from build123d import *

# Parameters (mm, degrees)
BOSS_EXTRUDE2_DEPTH   = 12.7
BOSS_EXTRUDE2_2_DEPTH = 12.7
SKETCH2_7_W           = 239.064376672
SKETCH2_7_H           = 153.94029831
BOSS_EXTRUDE3_DEPTH   = 12.7
SKETCH2_8_R           = 5.08
SKETCH2_8_R_2         = 3.81
BOSS_EXTRUDE4_DEPTH   = 50.8


with BuildPart() as part:
    # Sketch2 → Boss-Extrude2 (new body)
    with BuildSketch(Plane.XY):
        Polygon((-103.331182916, 71.628), (103.331182916, 71.628), (98.251182916, 76.708), (-98.251182916, 76.708), align=None)
    extrude(amount=BOSS_EXTRUDE2_DEPTH)



with BuildPart() as body_2:
    # Sketch2 → Boss-Extrude2 2 (new body)
    with BuildSketch(Plane.XY):
        Polygon((103.331182916, 107.188), (98.251182916, 102.108), (-98.251182916, 102.108), (-103.331182916, 107.188), align=None)
    extrude(amount=BOSS_EXTRUDE2_2_DEPTH)


with BuildPart() as part_1:
    add(part.part)

    add(body_2.part)  # Boss-Extrude3 merges body 2
    # Sketch2_7 → Boss-Extrude3 (add)
    with BuildSketch(Plane.XY):
        with Locations((0, 44.704)):
            Rectangle(SKETCH2_7_W, SKETCH2_7_H)
    extrude(amount=-BOSS_EXTRUDE3_DEPTH)

    # Sketch2_8 → Boss-Extrude4 (add)
    with BuildSketch(Plane.XY):
        with Locations((21.333013583, 41.868396572)):
            Circle(SKETCH2_8_R)
        Circle(SKETCH2_8_R_2)
    extrude(amount=BOSS_EXTRUDE4_DEPTH)


solid = part_1.part
Geometry check sheet. Reference: the model listing, model coordinates, mm. A direction names the side the tool comes from. Round coordinates to 2 decimals unless told otherwise and drop trailing zeros. Loops run counter-clockwise (first coordinate to the right, second up) from the corner with the lowest first, then second, coordinate; pieces in that order, holes last. Notation, with made-up numbers: (15, 10) -> (45, 10) arc R19 ccw to (45, 16) -> close; hole circle Ø1 at (-26, 40.5). An arc over 180 degrees is marked (long way). Answer as a JSON object with one key per item and string values. Group by question number.
Item 1: Cross-section at A-A, the plane x = -86. Record the cut outline in (y, z).
Item 2: Cross-section at B-B, the plane y = 0. Record the cut outline in (x, z), plus the area to 3 significant figures.
Item 3: Set-up check for faces 1 (the face through (100.83, 74.13, 6.26)), 2 (the face through (-100.756, 104.612, 6.261)), 3 (the face through (-1, 74, 12.7)), 4 (the face through (-0.83, -3.72, 25.04)), 5 (the face through (-1, 71.628, 6)): record each of +Z, -Z, +X, -X, +Y, -Y from which the full face is reachable in a straight line by a thin tool's end or side.
Item 4: Release check for a two-part mould opening along Y. For faces 6 (the face through (1, 105, 12.7)), 7 (the face through (100.827, 104.684, 6.261)), 8 (the face through (-2, -32.266, -6)) record: pulls with the +Y half, pulls with the -Y half, needs draft (parallel to the pull), parting line crosses it, or undercut.
Item 5: Cross-section at D-D, the plane x = 0. Record the cut outline in (y, z).
Item 6: Cross-section at C-C, the plane z = 6.5. Record the cut outline in (x, y).
Item 7: Depth check by flat-ended pin: pin 1 Ø6.5 at (x, z) = (4.5, 6) entering from +Y; pin 2 Ø6.5 at (x, z) = (25.5, 8) entering from -Y; pin 3 Ø2.5 at (x, y) = (-8, 105.5) entering from +Z; pin 4 Ø6 at (y, z) = (-7, 28) entering from -X. Enter the tip coordinate at first touch or a pass-through.
Item 8: Thickness scan on line 1 along Y through (x, z) = (-3.5, 2); line 2 along X through (y, z) = (0.5, 32); line 3 along Z through (x, y) = (92, 47). Record the ranges inside material, lowest first.
Determined:
{
 "1": {"outline": "(-32.27, -12.7) -> (121.67, -12.7) -> (121.67, 0) -> (107.19, 0) -> (107.19, 12.7) -> (102.11, 12.7) -> (102.11, 0) -> (76.71, 0) -> (76.71, 12.7) -> (71.63, 12.7) -> (71.63, 0) -> (-32.27, 0) -> close"},
 "2": {"outline": "(-119.53, -12.7) -> (119.53, -12.7) -> (119.53, 0) -> (3.81, 0) -> (3.81, 50.8) -> (-3.81, 50.8) -> (-3.81, 0) -> (-119.53, 0) -> close", "area": "3,420 mm²"},
 "3": {"face 1": "+Z, +X", "face 2": "+Z, -X", "face 3": "+Z, +X, -X, +Y", "face 4": "+Z", "face 5": "+Z, +X, -X"},
 "4": {"face 6": "needs draft", "face 7": "undercut", "face 8": "pulls with the -Y half"},
 "5": {"outline": "(-32.27, -12.7) -> (121.67, -12.7) -> (121.67, 0) -> (107.19, 0) -> (107.19, 12.7) -> (102.11, 12.7) -> (102.11, 0) -> (76.71, 0) -> (76.71, 12.7) -> (71.63, 12.7) -> (71.63, 0) -> (3.81, 0) -> (3.81, 50.8) -> (-3.81, 50.8) -> (-3.81, 0) -> (-32.27, 0) -> close"},
 "6": {"outline": "(-103.33, 71.63) -> (103.33, 71.63) -> (98.25, 76.71) -> (-98.25, 76.71) -> close; (-103.33, 107.19) -> (-98.25, 102.11) -> (98.25, 102.11) -> (103.33, 107.19) -> close; circle Ø7.62 at (0, 0); circle Ø10.16 at (21.33, 41.87)"},
 "7": {"pin 1": "stops at y = 107.19", "pin 2": "stops at y = 36.87", "pin 3": "stops at z = 12.7", "pin 4": "passes through"},
 "8": {"line 1": "y = -1.51 to 1.51, 71.63 to 76.71, 102.11 to 107.19", "line 2": "x = -3.78 to 3.78", "line 3": "z = -12.7 to 0"}
}
